Could you check a few things on this model? Use its own coordinates, in mm. A direction names the side the tool comes from. Round coordinates to 2 decimals unless told otherwise and drop trailing zeros. Loops run counter-clockwise (first coordinate to the right, second up) from the corner with the lowest first, then second, coordinate; pieces in that order, holes last. Notation, with made-up numbers: (-37, -25.75) -> (-28, -25.75) arc R15 cw to (-28, -14.75) -> close; hole circle Ø4 at (86.25, 36.5). An arc over 180 degrees is marked (long way). Put each result on its own line as item: value. Start each with the question number.
1. I'm going to push flat-ended pins straight in: P1, Ø1.9, axis at y = -2.5, z = 19, coming from the -X side; P2, Ø1.5, axis at y = -3, z = 18, coming from the -X side; P3, Ø3, axis at x = 18, y = -1.5, coming from the -Z side. Where does each tip first touch, or does it pass through?
2. Which directions (+Z, -Z, +X, -X, +Y, -Y) give clear straight access to the entire face, cutting with the end or side of a thin tool? Please do faces 4 (the flat face through (32.6, -2.5, 13.5)), 5 (the cylindrical face through (79.1, -2.5, 10.4)), 6 (the flat face through (-32, -3, 18.198)), 7 (the flat face through (-11.408, -2.504, 11.886)).
3. If we mould it in two halves opening along Z, with no side actions, what happens to faces 1 (the flat face through (1.12, -2.5, 26.1)), 2 (the flat face through (-20.16, -2.5, 15.77)), 3 (the flat face through (-28.144, -2.504, 36.163))? For each: pulls with the +Z half, pulls with the -Z half, needs draft (parallel to the pull), parting line crosses it, or undercut.
4. Imagine slicing it at A-A, the plane y = -2.8. Count the separate pieces of the cut face and the enclosed holes in it, and give its area (3 significant figures).
5. Imagine slicing it at B-B, the plane x = -39. Please give me the cut outline in (y, z), and give its area (3 significant figures).
6. I need wall thicknesses on line 1 (X direction, y = -2, z = 26.5); line 2 (Z direction, x = -0.5, y = -4.4); line 3 (Z direction, x = 31, y = -0.7). Which ranges of each line are inside material? Lowest first, please. Write a range as [from, to].
```python
from build123d import *

# Parameters (mm, degrees)
F1_DEPTH = 5.08


with BuildPart() as f1:
    # F0 (on Front) → F1 (new body)
    with BuildSketch(Plane.XZ):
        with BuildLine():
            Line((-40.275556, 44.046157), (-47.404758, 34.581525))
            ThreePointArc((-47.404758, 34.581525), (-48.669842, 30.357517), (-46.879273, 26.328058))
            Line((-46.879273, 26.328058), (-40.821373, 20.114827))
            ThreePointArc((-40.821373, 20.114827), (-38.741891, 18.696625), (-36.274772, 18.197764))
            Line((-36.274772, 18.197764), (-26.811405, 18.197764))
            ThreePointArc((-26.811405, 18.197764), (-25.449181, 18.049928), (-24.150386, 17.613306))
            Line((-24.150386, 17.613306), (-16.054588, 13.876783))
            Line((-16.054588, 13.876783), (-13.685921, 16.563832))
            Line((-13.685921, 16.563832), (-10.083565, 13.38831))
            Line((-10.083565, 13.38831), (-12.769917, 10.340875))
            Line((-12.769917, 10.340875), (-10.570144, 4.47481))
            ThreePointArc((-10.570144, 4.47481), (-10.228729, 3.136696), (-10.184672, 1.756416))
            Line((-10.184672, 1.756416), (-11.142575, -10.651773))
            ThreePointArc((-11.142575, -10.651773), (-9.914032, -14.920187), (-6.188922, -17.339322))
            Line((-6.188922, -17.339322), (3.625042, -19.520204))
            Line((3.625042, -19.520204), (24.356571, -24.127213))
            ThreePointArc((24.356571, -24.127213), (32.617279, -24.582682), (40.58616, -22.359246))
            Line((40.58616, -22.359246), (54.85313, -15.717725))
            ThreePointArc((54.85313, -15.717725), (59.411476, -12.982062), (63.300546, -9.357493))
            Line((63.300546, -9.357493), (71.362269, -0.086524))
            ThreePointArc((71.362269, -0.086524), (71.438277, -0.000693), (71.515821, 0.083752))
            Line((71.515821, 0.083752), (77.39452, 6.370687))
            ThreePointArc((77.39452, 6.370687), (79.101388, 10.457233), (77.721958, 14.66561))
            Line((77.721958, 14.66561), (74.67214, 18.491938))
            ThreePointArc((74.67214, 18.491938), (73.070176, 19.919962), (71.084022, 20.732817))
            Line((71.084022, 20.732817), (55.460665, 24.204676))
            ThreePointArc((55.460665, 24.204676), (52.678779, 24.507072), (49.898197, 24.192908))
            Line((49.898197, 24.192908), (30.802289, 19.864502))
            ThreePointArc((30.802289, 19.864502), (22.647473, 19.363428), (14.755452, 21.477216))
            Line((14.755452, 21.477216), (4.972792, 25.88382))
            ThreePointArc((4.972792, 25.88382), (3.570361, 26.568119), (2.212597, 27.337246))
            Line((2.212597, 27.337246), (0, 24.827245))
            Line((0, 24.827245), (-3.602356, 28.002767))
            Line((-3.602356, 28.002767), (-1.648816, 30.21889))
            ThreePointArc((-1.648816, 30.21889), (-2.65924, 31.186265), (-3.614876, 32.207799))
            Line((-3.614876, 32.207799), (-18.335917, 48.839203))
            ThreePointArc((-18.335917, 48.839203), (-19.867203, 50.101377), (-21.713309, 50.82926))
            Line((-21.713309, 50.82926), (-29.24698, 52.50341))
            ThreePointArc((-29.24698, 52.50341), (-32.821418, 52.262474), (-35.696574, 50.125153))
            Line((-35.696574, 50.125153), (-37.694322, 47.472969))
            Line((-37.694322, 47.472969), (-28.918262, 39.736762))
            Line((-28.918262, 39.736762), (-31.746839, 36.527986))
            Line((-31.746839, 36.527986), (-40.275556, 44.046157))
        make_face()
        with BuildLine():
            ThreePointArc((-4.225081, -13.529201), (-3.944831, -8.312931), (0.905035, -6.372102))
            Line((0.905035, -6.372102), (-3.15545, -12.829451))
            Line((-3.15545, -12.829451), (-4.225081, -13.529201))
        make_face(mode=Mode.SUBTRACT)
        with BuildLine():
            ThreePointArc((4.845113, -10.854332), (2.657107, -15.202162), (-2.203116, -15.465267))
            Line((-2.203116, -15.465267), (4.845113, -10.854332))
        make_face(mode=Mode.SUBTRACT)
        with BuildLine():
            ThreePointArc((2.641534, -7.068762), (3.312281, -7.592883), (3.881143, -8.226128))
            Line((3.881143, -8.226128), (0.53884, -10.412655))
            Line((0.53884, -10.412655), (2.641534, -7.068762))
        make_face(mode=Mode.SUBTRACT)
        with BuildLine():
            Line((8.424729, -8.512556), (14.443013, -4.575408))
            Line((14.443013, -4.575408), (15.546219, -10.843349))
            ThreePointArc((15.546219, -10.843349), (11.807481, -10.221791), (8.424729, -8.512556))
        make_face(mode=Mode.SUBTRACT)
        with BuildLine():
            Line((4.550004, -4.03374), (12.205012, 8.139946))
            Line((12.205012, 8.139946), (13.928658, -1.653066))
            Line((13.928658, -1.653066), (6.326088, -6.62665))
            ThreePointArc((6.326088, -6.62665), (5.356567, -5.386006), (4.550004, -4.03374))
        make_face(mode=Mode.SUBTRACT)
        with BuildLine():
            ThreePointArc((3.698579, -1.929555), (4.451633, 7.252294), (11.270996, 13.446624))
            Line((11.270996, 13.446624), (11.729453, 10.841867))
            Line((11.729453, 10.841867), (3.698579, -1.929555))
        make_face(mode=Mode.SUBTRACT)
        with BuildLine():
            ThreePointArc((24.562505, -16.508693), (23.048976, -20.625797), (18.664287, -20.500059))
            Line((18.664287, -20.500059), (24.562505, -16.508693))
        make_face(mode=Mode.SUBTRACT)
        with BuildLine():
            ThreePointArc((17.396329, -18.748226), (18.839082, -14.40465), (23.407693, -14.680293))
            Line((23.407693, -14.680293), (17.396329, -18.748226))
        make_face(mode=Mode.SUBTRACT)
        with BuildLine():
            ThreePointArc((28.408875, -11.295958), (27.6599, -7.249786), (29.281339, -3.467801))
            Line((29.281339, -3.467801), (33.01283, -8.18043))
            Line((33.01283, -8.18043), (28.408875, -11.295958))
        make_face(mode=Mode.SUBTRACT)
        with BuildLine():
            Line((29.683054, -13.043582), (34.358372, -9.879761))
            Line((34.358372, -9.879761), (37.916162, -14.373018))
            ThreePointArc((37.916162, -14.373018), (33.583819, -15.044666), (29.683054, -13.043582))
        make_face(mode=Mode.SUBTRACT)
        with BuildLine():
            ThreePointArc((44.73614, -14.067125), (44.771689, -8.173226), (50.616499, -7.413293))
            Line((50.616499, -7.413293), (44.73614, -14.067125))
        make_face(mode=Mode.SUBTRACT)
        with BuildLine():
            Line((39.879447, -12.907889), (31.157593, -1.892757))
            ThreePointArc((31.157593, -1.892757), (40.281312, -3.629113), (39.879447, -12.907889))
        make_face(mode=Mode.SUBTRACT)
        with BuildLine():
            ThreePointArc((51.917324, -8.746926), (51.486914, -14.107842), (46.21959, -15.194111))
            Line((46.21959, -15.194111), (51.917324, -8.746926))
        make_face(mode=Mode.SUBTRACT)
        with BuildLine():
            Line((17.489936, -10.717827), (15.603516, 0))
            Line((15.603516, 0), (23.100192, 4.338584))
            Line((23.100192, 4.338584), (27.815175, -1.616132))
            ThreePointArc((27.815175, -1.616132), (24.011433, -7.708531), (17.489936, -10.717827))
        make_face(mode=Mode.SUBTRACT)
        with BuildLine():
            Line((28.262959, 1.762977), (25.24207, 5.578162))
            Line((25.24207, 5.578162), (27.217829, 6.721602))
            ThreePointArc((27.217829, 6.721602), (27.993249, 4.295584), (28.262959, 1.762977))
        make_face(mode=Mode.SUBTRACT)
        with BuildLine():
            ThreePointArc((13.140761, 13.992305), (20.017468, 13.496749), (25.594964, 9.443823))
            Line((25.594964, 9.443823), (15.018651, 3.322948))
            Line((15.018651, 3.322948), (13.140761, 13.992305))
        make_face(mode=Mode.SUBTRACT)
        with BuildLine():
            Line((30.93997, 8.875732), (39.47801, 6.432929))
            ThreePointArc((39.47801, 6.432929), (33.560944, 3.82119), (28.046584, 7.201231))
            Line((28.046584, 7.201231), (30.93997, 8.875732))
        make_face(mode=Mode.SUBTRACT)
        with BuildLine():
            Line((40.888753, 9.564819), (35.028014, 11.241624))
            Line((35.028014, 11.241624), (40.103703, 14.1791))
            ThreePointArc((40.103703, 14.1791), (40.895382, 11.939869), (40.888753, 9.564819))
        make_face(mode=Mode.SUBTRACT)
        with BuildLine():
            Line((46.789589, 7.876541), (43.188322, 8.906893))
            ThreePointArc((43.188322, 8.906893), (45.411398, 13.138456), (49.147954, 16.119453))
            Line((49.147954, 16.119453), (46.789589, 7.876541))
        make_face(mode=Mode.SUBTRACT)
        with BuildLine():
            Line((54.422703, -5.912002), (60.114638, 0.528621))
            Line((60.114638, 0.528621), (64.136762, -0.622142))
            ThreePointArc((64.136762, -0.622142), (59.948363, -4.494914), (54.422703, -5.912002))
        make_face(mode=Mode.SUBTRACT)
        with BuildLine():
            ThreePointArc((52.13659, -5.693258), (45.467392, -1.754529), (42.747289, 5.497562))
            Line((42.747289, 5.497562), (58.135606, 1.094838))
            Line((58.135606, 1.094838), (52.13659, -5.693258))
        make_face(mode=Mode.SUBTRACT)
        Polygon((53.247314, 6.028933), (48.331221, 7.435468), (49.497491, 11.511795), align=None, mode=Mode.SUBTRACT)
        with BuildLine():
            ThreePointArc((51.030518, 16.87), (62.563308, 14.002848), (65.565734, 2.504533))
            Line((65.565734, 2.504533), (55.861395, 5.281023))
            Line((55.861395, 5.281023), (50.117643, 13.679339))
            Line((50.117643, 13.679339), (51.030518, 16.87))
        make_face(mode=Mode.SUBTRACT)
        Polygon((-20.639595, 26.73681), (-29.538747, 34.581525), (-26.71017, 37.790301), (-17.811018, 29.945587), align=None, mode=Mode.SUBTRACT)
        Polygon((-6.20836, 17.784396), (-8.572314, 15.102694), (-12.17467, 18.278216), (-11.680279, 18.83906), (-13.1406, 20.126352), (-6.20836, 20.126352), align=None, mode=Mode.SUBTRACT)
        Polygon((-11.416613, 24.308838), (-8.851702, 22.047837), (-6.20836, 25.04648), (-6.20836, 21.415438), (-11.416613, 21.415438), align=None, mode=Mode.SUBTRACT)
        Polygon((-4.286453, 19.964633), (-4.286453, 25.283757), (-1.647903, 22.957841), align=None, mode=Mode.SUBTRACT)
        Polygon((-14.602957, 21.415438), (-18.15631, 24.547764), (-15.327734, 27.75654), (-12.835704, 25.559785), (-12.835704, 21.415438), align=None, mode=Mode.SUBTRACT)
        with BuildLine():
            Line((37.897688, 16.563832), (27.077917, 10.302059))
            ThreePointArc((27.077917, 10.302059), (30.53882, 16.800609), (37.897688, 16.563832))
        make_face(mode=Mode.SUBTRACT)
    extrude(amount=F1_DEPTH)


solid = f1.part
```
Entries:
1. P1: x = -40.65
1. P2: x = -38.86
1. P3: z = -23.05
2. face 4: +Y, -Y
2. face 5: +X, +Y, -Y
2. face 6: -Z, -X, +Y, -Y
2. face 7: -X, +Y, -Y
3. face 1: pulls with the +Z half
3. face 2: pulls with the -Z half
3. face 3: undercut
4. separate pieces: 1
4. enclosed holes: 29
4. area: 3,530 mm^2
5. outline: (-5.08, 18.81) -> (0, 18.81) -> (0, 42.92) -> (-5.08, 42.92) -> close
5. area: 122 mm^2
6. line 1: [-47.04, -16.44], [-13.9, -1.9], [1.47, 3.7]
6. line 2: [-18.6, -15.97], [-14.35, -8.61], [-6.31, 25.27]
6. line 3: [-24.71, -14.09], [-12.15, -9.54], [-5.64, 4.5], [8.86, 12.57], [17.04, 19.91]
